Here's the drawing with two shaded views (mm, measured from the low corner). I have some questions. Coordinates: 2 decimals unless noted, no trailing zeros. Write each loop counter-clockwise with the first axis right and the second up, starting at its lowest first coordinate (ties: lowest second). Pieces come first, ordered by that corner, then holes.
Item 1: For P1, Ø1.5, axis at x = 57, z = 1, coming from the -Y side; P2, Ø3, axis at x = 53.5, z = 4, coming from the +Y side; P3, Ø1.5, axis at x = 37, y = 1.5, coming from the -Z side, each with a flat end and sliding along its axis, tell me the tip position at first contact or that it passes through.
Item 2: I want a section at A-A on x = 89. Please give me the cut outline in (y, z) (1 decimal).
Item 3: I want a section at B-B on z = 4.3. Please give me the cut outline in (x, y) (1 decimal).
Item 4: If I drill on probe 1 along Z at (x, y) = (88, 5.75) (1 decimal); probe 2 along Y at (x, z) = (19, 4.8) (1 decimal); probe 3 along Y at (x, z) = (39, 0.5) (1 decimal), over which ranges is the centre line in solid material (lowest first)?
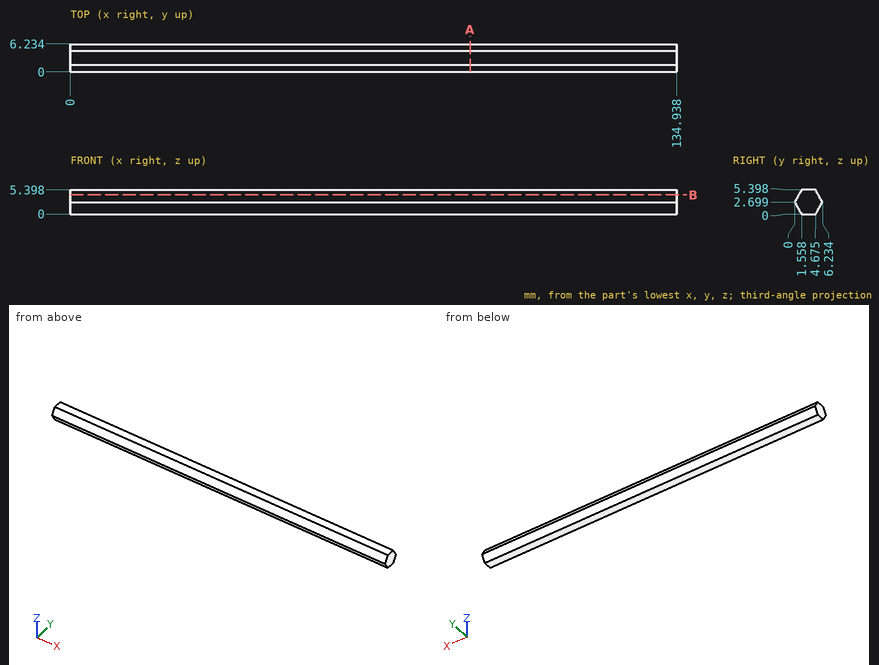
Response values:
1. P1: stops at y = 0.55
1. P2: stops at y = 6.23
1. P3: stops at z = 0
2. outline: (0, 2.7) - (1.6, 0) - (4.7, 0) - (6.2, 2.7) - (4.7, 5.4) - (1.6, 5.4) - close
3. outline: (0, 0.9) - (134.9, 0.9) - (134.9, 5.3) - (0, 5.3) - close
4. probe 1: z = 1.9 to 3.5
4. probe 2: y = 1.2 to 5
4. probe 3: y = 1.3 to 5
